from build123d import *

# Parameters (mm, degrees)
BASE_FLANGE1_DEPTH  = 2
CUT_EXTRUDE13_DEPTH = 10
BOSS_EXTRUDE4_DEPTH = 2
BOSS_EXTRUDE5_START = -2
BOSS_EXTRUDE5_DEPTH = 2
SKETCH18_R          = 6
CUT_EXTRUDE14_DEPTH = 87.861941803
SKETCH19_R          = 3
CUT_EXTRUDE15_DEPTH = 86.495161894


# Sheet-metal steps are written as plain solids
with BuildPart() as part:
    # Sketch2 → Base-Flange1 (new body)
    with BuildSketch(Plane(origin=(0, 0, 0), x_dir=(1, 0, 0), z_dir=(0, 1, 0))):
        with BuildLine():
            Line((20, 27.099918438), (20, -57.900081562))
            ThreePointArc((20, -57.900081562), (0, -77.900081562), (-20, -57.900081562))
            Line((-20, -57.900081562), (-20, 27.099918438))
            ThreePointArc((-20, 27.099918438), (0, 47.099918438), (20, 27.099918438))
        make_face()
    extrude(amount=-BASE_FLANGE1_DEPTH)

    # Sketch9 → Cut-Extrude13 (cut)
    with BuildSketch(Plane(origin=(0, 0, 0), x_dir=(1, 0, 0), z_dir=(0, 1, 0))):
        with BuildLine():
            Line((9, 1.599918438), (-9, 1.599918438))
            Line((-9, 1.599918438), (-9, 19.599918438))
            ThreePointArc((-9, 19.599918438), (0, 28.599918438), (9, 19.599918438))
            Line((9, 19.599918438), (9, 1.599918438))
        make_face()
        with BuildLine():
            Line((-9, -32.400081562), (9, -32.400081562))
            Line((9, -32.400081562), (9, -50.400081562))
            ThreePointArc((9, -50.400081562), (0, -59.400081562), (-9, -50.400081562))
            Line((-9, -50.400081562), (-9, -32.400081562))
        make_face()
    extrude(amount=-CUT_EXTRUDE13_DEPTH, mode=Mode.SUBTRACT)

    # Sketch16 → Boss-Extrude4 (add)
    with BuildSketch(Plane.XY.offset(31)):
        with BuildLine():
            Line((-9, -2), (-9, 18))
            ThreePointArc((-9, 18), (0, 27), (9, 18))
            Line((9, 18), (9, -2))
            Line((9, -2), (-9, -2))
        make_face()
    extrude(amount=BOSS_EXTRUDE4_DEPTH)

    # Sketch17 → Boss-Extrude5 (add)
    with BuildSketch(Plane.XY.offset(-1.985).offset(BOSS_EXTRUDE5_START)):
        with BuildLine():
            Line((9, -2), (9, 18))
            ThreePointArc((9, 18), (0, 27), (-9, 18))
            Line((-9, 18), (-9, -2))
            Line((-9, -2), (9, -2))
        make_face()
    extrude(amount=BOSS_EXTRUDE5_DEPTH)

    # Sketch18 → Cut-Extrude14 (cut, through all)
    with BuildSketch(Plane.XY.offset(33)):
        with Locations((0, 18)):
            Circle(SKETCH18_R)
    extrude(amount=-CUT_EXTRUDE14_DEPTH, mode=Mode.SUBTRACT)

    # Sketch19 → Cut-Extrude15 (cut, through all)
    with BuildSketch(Plane.XZ.offset(2)):
        with Locations(Location((0, 69.400081562, 0), (0, 0, 270))):
            Circle(SKETCH19_R)
        with Locations(Location((0, -38.599918438, 0), (0, 0, 270))):
            Circle(SKETCH19_R)
    extrude(amount=-CUT_EXTRUDE15_DEPTH, mode=Mode.SUBTRACT)


solid = part.part
Check sheet for the modelled part. Datum: model origin and axes. Units: mm. A direction names the side the tool comes from. Round coordinates to 2 decimals unless told otherwise and drop trailing zeros. Order: outer loops, then holes, each group sorted by start corner. A loop starts at its lowest first (then second) coordinate and runs counter-clockwise, first axis right, second up. Notation, with made-up numbers: M 25,-4 L 37,-4 A21 cw 37,32 Z; hole C -19.75,31.25 d5. An arc over 180 degrees is marked long. One line per item, written item: value. Start each with the question number.
1. Release check for a two-part mould opening along Z. For faces 1 (the cylindrical face through (-6, 18, 32)), 2 (the cylindrical face through (0.198, -0.986, 59.398)), 3 (the cylindrical face through (0.1, -1, 72.4)), 4 (the cylindrical face through (-0.44, -0.986, -47.095)) record: released by +Z, released by -Z, zero draft, split by the parting line, or undercut.
2. Gauge pin test, flat ends, axial feed: P1, Ø7, axis at x = 0, z = 69.4, coming from the +Y side; P2, Ø2, axis at y = 13, z = -3.5, coming from the -X side; P3, Ø8, axis at x = 0, z = -38.6, coming from the -Y side; P4, Ø1.6, axis at y = 8.5, z = 32, coming from the +X side. Record the tip position at first contact, or that the pin passes through.
3. Access from +Z, -Z, +X, -X, +Y, -Y to the whole of each face (thin tool, end or side, straight path). Record for faces 5 (the flat face through (0, 11, 31)), 6 (the cylindrical face through (0, 27, -3)), 7 (the flat face through (0, 9, -1.985)).
4. Scan lines: line 1 along Z through (x, y) = (-8, 9.75) (3 decimals); line 2 along Y through (x, z) = (-6, -39.5). Record each from-to range of solid material in increasing order.
5. Section check B-B on x = 0. Give the number of separate pieces and of enclosed holes in the cut face, and give its area (3 significant figures).
6. Section check A-A on z = -15.5. Enter the section's corners in (x, y).
7. Section check C-C on y = 7.5. Enter the section's corners in (x, z) (3 decimals).
8. Section check D-D on y = 20.25. Enter the section's corners in (x, z) (3 decimals), and give its area (3 significant figures).
Results found:
1. face 1: zero draft
1. face 2: undercut
1. face 3: undercut
1. face 4: released by -Z
2. P1: y = 0
2. P2: x = -9
2. P3: y = -2
2. P4: x = 9
3. face 5: +X, -X, +Y
3. face 6: +Z, -Z, +Y
3. face 7: +Y, -Y
4. line 1: -3.985 to -1.985, 31 to 33
4. line 2: -2 to 0
5. separate pieces: 8
5. enclosed holes: 0
5. area: 183 mm^2
6. outline: M -20,-2 L -9,-2 L -9,0 L -20,0 Z; M 9,-2 L 20,-2 L 20,0 L 9,0 Z
7. outline: M -9,-3.985 L 9,-3.985 L 9,-1.985 L -9,-1.985 Z; M -9,31 L 9,31 L 9,33 L -9,33 Z
8. outline: M -8.714,-3.985 L -5.562,-3.985 L -5.562,-1.985 L -8.714,-1.985 Z; M -8.714,31 L -5.562,31 L -5.562,33 L -8.714,33 Z; M 5.562,-3.985 L 8.714,-3.985 L 8.714,-1.985 L 5.562,-1.985 Z; M 5.562,31 L 8.714,31 L 8.714,33 L 5.562,33 Z
8. area: 25.2 mm^2
